from build123d import *

# Parameters (mm, degrees)
EXTRUDE_1_DEPTH     = 27.5
SKETCH_2_R          = 1.5
CUT_EXTRUDE_1_DEPTH = 3
SKETCH_3_R          = 0.75
CUT_EXTRUDE_3_DEPTH = 3
REVOLVE_1_ANGLE     = 270


with BuildPart() as part:
    # 草图1 → 凸台-拉伸1 (new, symmetric)
    with BuildSketch(Plane(origin=(0, 0, 0), x_dir=(1, 0, 0), z_dir=(0, 1, 0))):
        Polygon((5.882352941, 27.284313725), (25.882352941, 27.284313725), (25.882352941, -27.715686275), (22.882352941, -27.715686275), (22.882352941, 24.284313725), (5.882352941, 24.284313725), align=None)
    extrude(amount=EXTRUDE_1_DEPTH, both=True)

    # 草图2 → 切除-拉伸1 (cut)
    with BuildSketch(Plane(origin=(0, 0, -27.284313725), x_dir=(-1, 0, 0), z_dir=(0, 0, -1))):
        with Locations((-13.382352941, 10)):
            Circle(SKETCH_2_R)
        with Locations((-13.382352941, -10)):
            Circle(SKETCH_2_R)
    extrude(amount=-CUT_EXTRUDE_1_DEPTH, mode=Mode.SUBTRACT)

    # 草图3 → 切除-拉伸3 (cut)
    with BuildSketch(Plane(origin=(25.882352941, 0, 0), x_dir=(0, 0, -1), z_dir=(1, 0, 0))):
        with BuildLine():
            ThreePointArc((-19.394463571, 5.743970558), (-21.414171084, 0), (-19.394463571, -5.743970558))
            Line((-19.394463571, -5.743970558), (-18.726093915, -6.48959236))
            ThreePointArc((-18.726093915, -6.48959236), (-12.715686275, -21), (-6.705278634, -6.48959236))
            Line((-6.705278634, -6.48959236), (-6.036908978, -5.743970558))
            ThreePointArc((-6.036908978, -5.743970558), (-4.017201465, 0), (-6.036908978, 5.743970558))
            Line((-6.036908978, 5.743970558), (-6.705278634, 6.48959236))
            ThreePointArc((-6.705278634, 6.48959236), (-12.715686275, 21), (-18.726093915, 6.48959236))
            Line((-18.726093915, 6.48959236), (-19.394463571, 5.743970558))
        make_face()
        with Locations((-4.215686275, -21)):
            Circle(SKETCH_3_R)
        with Locations((-21.215686275, -21)):
            Circle(SKETCH_3_R)
        with Locations((-4.215686275, 21)):
            Circle(SKETCH_3_R)
        with Locations((-21.215686275, 21)):
            Circle(SKETCH_3_R)
    extrude(amount=-CUT_EXTRUDE_3_DEPTH, mode=Mode.SUBTRACT)

    # 草图5 → 旋转1 (revolve, symmetric)
    with BuildSketch(Plane(origin=(0, 0, 12.715686275), x_dir=(0, -1, 0), z_dir=(0, 0, 1))) as revolve_1_sk:
        Polygon((-22, 25.882352941), (-24.5, 32.882352941), (-23.5, 32.882352941), (-21, 25.882352941), align=None)
    revolve_1 = revolve(axis=Axis((32.882352941, 12.5, 12.715686275), (-1, 0, 0)), revolution_arc=REVOLVE_1_ANGLE / 2)
    revolve_1 = revolve_1 + revolve(revolve_1_sk.sketch, axis=Axis((32.882352941, 12.5, 12.715686275), (1, 0, 0)), revolution_arc=REVOLVE_1_ANGLE / 2)

    # 镜向1: 旋转1 across plane
    add(revolve_1.mirror(Plane.ZX))


solid = part.part
Read the model definition and answer for the solid it produces. Units are mm, in the model's axes. A direction names the side the tool comes from. Give positions to 0.01 mm unless a question says otherwise; leave off trailing zeros. Write each loop counter-clockwise with the first axis right and the second up, starting at its lowest first coordinate (ties: lowest second). Pieces come first, ordered by that corner, then holes. Notation, with made-up numbers: (-21, -38) -> (18, -38) arc R16 cw to (18, -24) -> close; hole circle Ø11 at (59, 4). An arc over 180 degrees is marked (long way). Answer as a JSON object with one key per item and string values. Group by question number.
1) Find section D-D (x = 19.5). Write down the section's boundary in (y, z).
2) Find section C-C (z = -15). Write down the section's boundary in (x, y), and give its area (3 significant figures).
3) Each of these flat-tipped pins is pushed along its axis until it touches: P1, Ø5, axis at y = 12.5, z = 4, coming from the +X side; P2, Ø2.5, axis at x = 13.38, y = 10, coming from the -Z side; P3, Ø16.5, axis at y = 1.5, z = -11.5, coming from the +X side; P4, Ø1.7, axis at y = 21, z = 21.22, coming from the -X side. Where does it stop, or does it pass through?
4) Find section B-B (y = 12.5). Write down the section's boundary in (x, z).
5) Consider L1, parallel to Z at x = 24, y = 6.5; L2, parallel to Z at x = 23.85, y = 12.5; L3, parallel to Y at x = 23.25, z = 12.5. Determine where each line is inside the solid, lowest interval first. Write a range as from..to.
6) Find section A-A (y = -1). Write down the section's boundary in (x, z).
7) The mould has two halves that part along Y. Classify faces 4 (the flat face through (23.3, 27.5, -6)), 5 (the flat face through (16, 0, -27.284)), 6 (the cylindrical face through (24.4, 20.27, 4.38)): +Y half, -Y half, draft (parallel to the pull), parting line (faces both ways), or undercut.
8) A tool of negligible diameter and unlimited length cuts with its end or side. For faces 1 (the cylindrical face through (24.4, -21.73, 4.38)), 2 (the flat face through (29.139, -5.258, 5.474)), 3 (the flat face through (15, 0, -24.284)), from which of +Z, -Z, +X, -X, +Y, -Y can it reach the whole face along a straight path? Write none if from no direction.
Values follow:
{
 "1": {"outline": "(-27.5, -27.28) -> (27.5, -27.28) -> (27.5, -24.28) -> (-27.5, -24.28) -> close"},
 "2": {"outline": "(22.88, -27.5) -> (25.88, -27.5) -> (25.88, 27.5) -> (22.88, 27.5) -> close", "area": "165 mm2"},
 "3": {"P1": "stops at x = 32.88", "P2": "passes through", "P3": "stops at x = 25.88", "P4": "stops at x = 22.88"},
 "4": {"outline": "(5.88, -27.28) -> (25.88, -27.28) -> (25.88, 3.22) -> (32.88, 0.72) -> (32.88, 1.72) -> (25.88, 4.22) -> (22.88, 4.22) -> (22.88, -24.28) -> (5.88, -24.28) -> close; (22.88, 21.22) -> (25.88, 21.22) -> (32.88, 23.72) -> (32.88, 24.72) -> (25.88, 22.22) -> (25.88, 27.72) -> (22.88, 27.72) -> close"},
 "5": {"L1": "z = -27.28..6.69, 18.74..27.72", "L2": "z = -27.28..4.22, 21.22..27.72", "L3": "y = -27.5..-21, 21..27.5"},
 "6": {"outline": "(5.88, -27.28) -> (25.88, -27.28) -> (25.88, 4.07) -> (22.88, 4.07) -> (22.88, -24.28) -> (5.88, -24.28) -> close; (22.88, 21.36) -> (25.88, 21.36) -> (25.88, 27.72) -> (22.88, 27.72) -> close"},
 "7": {"face 4": "+Y half", "face 5": "draft", "face 6": "undercut"},
 "8": {"face 1": "-X", "face 2": "+X", "face 3": "+Z, -X, +Y, -Y"}
}
